Design review of the part built by this model. Coordinates are the model's own, in mm. Face numbers are marked on the shaded views. A direction names the side the tool comes from. Coordinates: 2 decimals unless noted, no trailing zeros. Order: outer loops, then holes, each group sorted by start corner. A loop starts at its lowest first (then second) coordinate and runs counter-clockwise, first axis right, second up.
from build123d import *

# Parameters (mm, degrees)
F0_W     = 132.888824
F0_H     = 64.624012
F1_DEPTH = 25.4
F2_W     = 15.473353
F2_H     = 27.002521
F3_DEPTH = 3.81
F4_R     = 1.62741
F5_DEPTH = 1.27
F7_DEPTH = 132.588


with BuildPart() as f1:
    # F0 (on Front) → F1 (new body, symmetric)
    with BuildSketch(Plane.XZ):
        Rectangle(F0_W, F0_H)
    extrude(amount=F1_DEPTH, both=True)

    # F2 (on face) → F3 (join)
    with BuildSketch(Plane.XZ.offset(25.4)):
        with Locations((-0.455099, -18.810745)):
            Rectangle(F2_W, F2_H)
    extrude(amount=F3_DEPTH)

    # F4 (on face) → F5 (join)
    with BuildSketch(Plane.XZ.offset(29.21)):
        with Locations((3.599366, -18.810746)):
            Circle(F4_R)
    extrude(amount=F5_DEPTH)

    # F6 (on face) → F7 (join)
    with BuildSketch(Plane(origin=(-66.444412, 0, 0), x_dir=(0, -1, 0), z_dir=(-1, 0, 0))):
        Polygon((25.4, 32.312006), (0, 55.370338), (-25.4, 32.312006), align=None)
    extrude(amount=-F7_DEPTH)


solid = f1.part
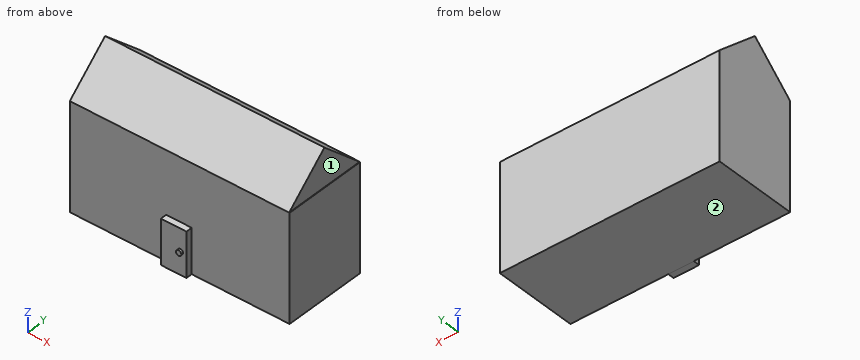
1. Add section A-A (z = -23.5). Give the boundary of the cut face in (x, y), and give its area (3 significant figures).
2. For the marked faces 1 and 2, list the 3-axis set-ups (+Z, -Z, +X, -X, +Y, -Y) from which the entire face can be reached by the end or side of a thin tool; tool diameter is ignored.
3. Add section C-C (y = -22). Give the boundary of the cut face in (x, z).
4. Add section D-D (x = 0.5). Give the boundary of the cut face in (y, z).
5. Add section B-B (x = -31.5). Give the boundary of the cut face in (y, z), and give its area (3 significant figures).
6. To check wall thickness, follow line 1 (Y direction, x = 32, z = -21); line 2 (Z direction, x = 13, y = -5.5); line 3 (Y direction, x = -6.5, z = -10.5). State the ranges of each line that lie inside material, in increasing order.
7. Insertion check: pin 1 (2 mm diameter, centred on x = -51, z = 28.5, fed in from -Y); pin 2 (4 mm diameter, centred on x = 0, y = -27, fed in from +Z); pin 3 (7.5 mm diameter, centred on x = -1, z = -18, fed in from -Y); pin 4 (4 mm diameter, centred on y = -27.5, z = -14.5, fed in from -X). Each pin has a flat end and moves straight along its axis. Give the tip position at first contact, or say it passes through.
Solution:
1. outline: (-66.44, -25.4) - (-8.19, -25.4) - (-8.19, -29.21) - (7.28, -29.21) - (7.28, -25.4) - (66.44, -25.4) - (66.44, 25.4) - (-66.44, 25.4) - close
1. area: 6,810 mm2
2. face 1: +Z, +X, +Y, -Y
2. face 2: -Z, +X, -X, +Y, -Y
3. outline: (-66.44, -32.31) - (66.44, -32.31) - (66.44, 32.31) - (66.14, 32.31) - (66.14, 35.4) - (-66.44, 35.4) - close
4. outline: (-29.21, -32.31) - (25.4, -32.31) - (25.4, 32.31) - (0, 55.37) - (-25.4, 32.31) - (-25.4, -5.31) - (-29.21, -5.31) - close
5. outline: (-25.4, -32.31) - (25.4, -32.31) - (25.4, 32.31) - (0, 55.37) - (-25.4, 32.31) - close
5. area: 3,870 mm2
6. line 1: y = -25.4 to 25.4
6. line 2: z = -32.31 to 50.38
6. line 3: y = -29.21 to 25.4
7. pin 1: stops at y = -25.4
7. pin 2: stops at z = 32.68
7. pin 3: stops at y = -30.48
7. pin 4: stops at x = -8.19
